Input: part model. Units: mm. Frame: model coordinates. Round coordinates to 2 decimals unless told otherwise and drop trailing zeros. Loops run counter-clockwise (first coordinate to the right, second up) from the corner with the lowest first, then second, coordinate; pieces in that order, holes last. Notation, with made-up numbers: (41.25, 83) - (52.25, 83) arc R9 cw to (52.25, 99) - close; hole circle Ø8 at (26.5, -40). An arc over 180 degrees is marked (long way). Use CSV: the item, a comma, the result in double quotes. Start each with the question number.
1. Cut plane B-B (y = -38.1). Return loops of the section in (x, z), and give its area (3 significant figures).
2. Material intervals for probe 1 along Y at (x, z) = (25.4, 1.75); probe 2 along Y at (x, z) = (-12.7, 1.8); probe 3 along Y at (x, z) = (25.4, 10.75), sorted ascending. Write a range as from..to.
3. Cut plane C-C (x = 12.7). Return loops of the section in (y, z).
4. Pin query (flat end, axial travel): P1, Ø3, axis at x = 25.4, y = -38.1, coming from the +Z side; P2, Ø14.5, axis at x = 12.7, y = -12.7, coming from the +Z side; P3, Ø5, axis at x = 27, y = -38, coming from the -Z side; P4, Ø9, axis at x = -13, y = -12.5, coming from the +Z side. Return the tip coordinate at first contact, or that it passes through.
5. Cut plane A-A (z = 1.75). Give the number of separate pieces and of enclosed holes in the cut face, and give its area (3 significant figures).
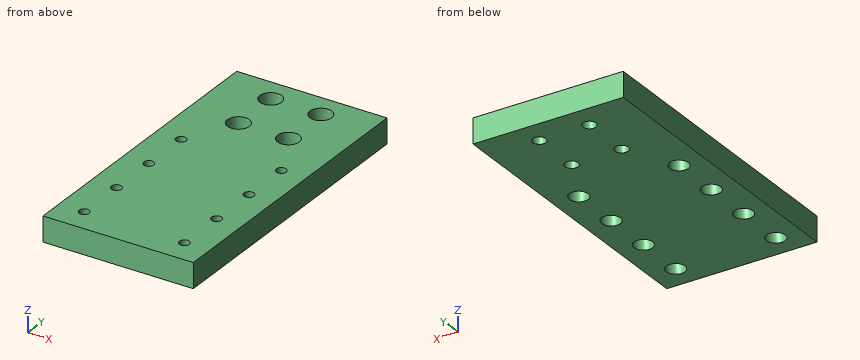
```python
from build123d import *

# Parameters (mm, degrees)
SKETCH1_W                                        = 76.2
SKETCH1_H                                        = 152.4
BOSS_EXTRUDE1_DEPTH                              = 12.7
CBORE_FOR_1_4_SOCKET_HEAD_CAP_SCREW1_D           = 6.7564
CBORE_FOR_1_4_SOCKET_HEAD_CAP_SCREW1_CBORE_D     = 11.1125
CBORE_FOR_1_4_SOCKET_HEAD_CAP_SCREW1_CBORE_DEPTH = 8.89
CBORE_FOR_10_SOCKET_HEAD_CAP_SCREW1_D            = 5.1054
CBORE_FOR_10_SOCKET_HEAD_CAP_SCREW1_CBORE_D      = 9.525
CBORE_FOR_10_SOCKET_HEAD_CAP_SCREW1_CBORE_DEPTH  = 7.366


with BuildPart() as part:
    # Sketch1 → Boss-Extrude1 (new body)
    with BuildSketch(Plane.XY):
        with Locations((0, -50.8)):
            Rectangle(SKETCH1_W, SKETCH1_H)
    extrude(amount=BOSS_EXTRUDE1_DEPTH)

    # CBORE for 1/4 Socket Head Cap Screw1 (through all)
    with Locations(Plane.XY.offset(12.7)):
        with Locations((-12.7, 12.7), (-12.7, -12.7), (12.7, -12.7), (12.7, 12.7)):
            CounterBoreHole(CBORE_FOR_1_4_SOCKET_HEAD_CAP_SCREW1_D / 2, CBORE_FOR_1_4_SOCKET_HEAD_CAP_SCREW1_CBORE_D / 2, CBORE_FOR_1_4_SOCKET_HEAD_CAP_SCREW1_CBORE_DEPTH)

    # CBORE for #10 Socket Head Cap Screw1 (through all)
    with Locations(Plane(origin=(0, 0, 0), x_dir=(-1, 0, 0), z_dir=(0, 0, -1))):
        with Locations((-25.4, -114.3), (25.4, -114.3), (25.4, -88.9), (25.4, -63.5), (25.4, -38.1), (-25.4, -88.9), (-25.4, -63.5), (-25.4, -38.1)):
            CounterBoreHole(CBORE_FOR_10_SOCKET_HEAD_CAP_SCREW1_D / 2, CBORE_FOR_10_SOCKET_HEAD_CAP_SCREW1_CBORE_D / 2, CBORE_FOR_10_SOCKET_HEAD_CAP_SCREW1_CBORE_DEPTH)


solid = part.part
```
Established:
1,outline,"(-38.1, 0) - (-30.16, 0) - (-30.16, 7.37) - (-27.95, 7.37) - (-27.95, 12.7) - (-38.1, 12.7) - close; (-22.85, 7.37) - (-20.64, 7.37) - (-20.64, 0) - (20.64, 0) - (20.64, 7.37) - (22.85, 7.37) - (22.85, 12.7) - (-22.85, 12.7) - close; (27.95, 7.37) - (30.16, 7.37) - (30.16, 0) - (38.1, 0) - (38.1, 12.7) - (27.95, 12.7) - close"
1,area,"773 mm2"
2,probe 1,"y = -127..-119.06, -109.54..-93.66, -84.14..-68.26, -58.74..-42.86, -33.34..25.4"
2,probe 2,"y = -127..-16.08, -9.32..9.32, 16.08..25.4"
2,probe 3,"y = -127..-116.85, -111.75..-91.45, -86.35..-66.05, -60.95..-40.65, -35.55..25.4"
3,outline,"(-127, 0) - (-16.08, 0) - (-16.08, 3.81) - (-18.26, 3.81) - (-18.26, 12.7) - (-127, 12.7) - close; (-9.32, 0) - (9.32, 0) - (9.32, 3.81) - (7.14, 3.81) - (7.14, 12.7) - (-7.14, 12.7) - (-7.14, 3.81) - (-9.32, 3.81) - close; (16.08, 0) - (25.4, 0) - (25.4, 12.7) - (18.26, 12.7) - (18.26, 3.81) - (16.08, 3.81) - close"
4,P1,"passes through"
4,P2,"stops at z = 12.7"
4,P3,"stops at z = 7.37"
4,P4,"stops at z = 3.81"
5,separate pieces,"1"
5,enclosed holes,"12"
5,area,"10,900 mm2"
